Design review of the part built by this model. Coordinates are the model's own, in mm. Face numbers are marked on the shaded views. A direction names the side the tool comes from. Give positions to 0.01 mm unless a question says otherwise; leave off trailing zeros. Loops run counter-clockwise (first coordinate to the right, second up) from the corner with the lowest first, then second, coordinate; pieces in that order, holes last. Notation, with made-up numbers: (-4, -32) - (48, -32) arc R18 cw to (48, 0) - close; hole circle Ø6 at (-15.5, -37.75). An arc over 180 degrees is marked (long way). Write each question's results on one line, items separated by ' | '.
Autodesk Inventor part; units mm, degrees
ref_plane "YZ Plane" through (0, 0, 0) normal (1, 0, 0) x (0, 1, 0)
ref_plane "XZ Plane" through (0, 0, 0) normal (0, 1, 0) x (-1, 0, 0)
ref_plane "XY Plane" through (0, 0, 0) normal (0, 0, 1) x (1, 0, 0)
sketch "Sketch1" plane through (0, 0, 0) normal (0, 1, 0) x (-1, 0, 0)
  line L0 (0, 0) -> (127, 0)
  line L1 (127, 0) -> (127, 118.999)
  line L2 (127, 118.999) -> (0, 118.999)
  line L3 (0, 118.999) -> (0, 0)
  dimension "d0" = 127
  dimension "d1" = 118.999
extrude "Plate1" add sketch "Sketch1" along normal blind 3.048
sketch "Sketch2" plane through (-123.952, 0, 118.999) normal (-1, 0, 0) x (0, -1, 0)
  line L0 (0, -118.999) -> (0, 0)
  line L1 (0, 0) -> (-25.4, 0)
  line L2 (-25.4, 0) -> (-25.4, -118.999)
  line L3 (-25.4, -118.999) -> (0, -118.999)
edge flange "Flange1" height 25.4 angle 90 thickness 3.048 bend radius 3.048 thickness toward (-1, 0, 0) relief tear relief width 3.048 relief depth 1.524 edges at (-127, 3.048, 59.4995) wall of the first edge with corners at (-123.952, 0, 0) (-123.952, 0, 118.999) (-123.952, 25.4, 118.999) (-123.952, 25.4, 0)
bend "Bend1"
corner "Corner1"
sketch "Sketch3" plane through (-3.048, 0, 0) normal (1, 0, 0) x (0, 1, 0)
  line L0 (0, 118.999) -> (0, 0)
  line L1 (0, 0) -> (25.4, 0)
  line L2 (25.4, 0) -> (25.4, 118.999)
  line L3 (25.4, 118.999) -> (0, 118.999)
edge flange "Flange2" height 25.4 angle 90 thickness 3.048 bend radius 3.048 thickness toward (1, 0, 0) relief tear relief width 3.048 relief depth 1.524 edges at (0, 3.048, 59.4995) wall of the first edge with corners at (-3.048, 0, 118.999) (-3.048, 0, 0) (-3.048, 25.4, 0) (-3.048, 25.4, 118.999)
bend "Bend2"
corner "Corner2"
sketch "Sketch4" plane through (0, 3.048, 0) normal (0, 1, 0) x (1, 0, 0)
  line L0 (-120.904, 0) -> (-6.096, 0)
  line L1 (-6.096, -118.999) -> (-120.904, -118.999)
  point P0 (0, 0)
  point P1 (-63.5, -99.949)
  point P2 (-63.5, -19.05)
  dimension "d23" = 19.05
  dimension "d24" = 19.05
hole "Hole1" at (-63.5, 3.048, 99.949) at (-63.5, 3.048, 19.05) direction (0, -1, 0) diameter 6.35 end through all
sketch "Sketch5" plane through (-127, 25.4, 0) normal (-1, 0, 0) x (0, 0, 1)
  line L0 (118.999, 0) -> (118.999, -19.304)
  line L1 (0, -19.304) -> (0, 0)
  line L2 (118.999, -25.4) -> (0, -25.4)
  point P0 (7.112, -12.7)
  point P1 (111.887, -12.7)
  dimension "d32" = 7.112
  dimension "d33" = 7.112
  dimension "d34" = 12.7
  dimension "d35" = 12.7
hole "Hole2" at (-127, 12.7, 7.112) at (-127, 12.7, 111.887) direction (1, 0, 0) diameter 4.2926 depth 1016 tip angle 118
equation "\"d30\" = Thickness"
equation "\"d3\" = BendReliefWidth"
equation "\"d4\" = BendReliefDepth"
equation "\"d5\" = MinimumRemnant"
equation "\"d6\" = BendRadius"
equation "\"d9\" = BendRadius"
equation "\"d10\" = CornerReliefSize"
equation "\"d11\" = GapSize"
equation "\"d12\" = JacobiRadiusSize"
equation "\"d13\" = BendReliefWidth"
equation "\"d14\" = BendReliefDepth"
equation "\"d15\" = MinimumRemnant"
equation "\"d16\" = BendRadius"
equation "\"d19\" = BendRadius"
equation "\"d20\" = CornerReliefSize"
equation "\"d21\" = GapSize"
equation "\"d22\" = JacobiRadiusSize"
equation "\"BendRadius\" = Thickness"
equation "\"BendReliefWidth\" = Thickness"
equation "\"BendReliefDepth\" = 0.5 * Thickness"
equation "\"CornerReliefSize\" = 4 * Thickness"
equation "\"MinimumRemnant\" = 2 * Thickness"
equation "\"TransitionRadius\" = BendRadius"
equation "\"JacobiRadiusSize\" = BendRadius"
equation "\"GapSize\" = Thickness"
equation "\"d2\" = BendRadius"
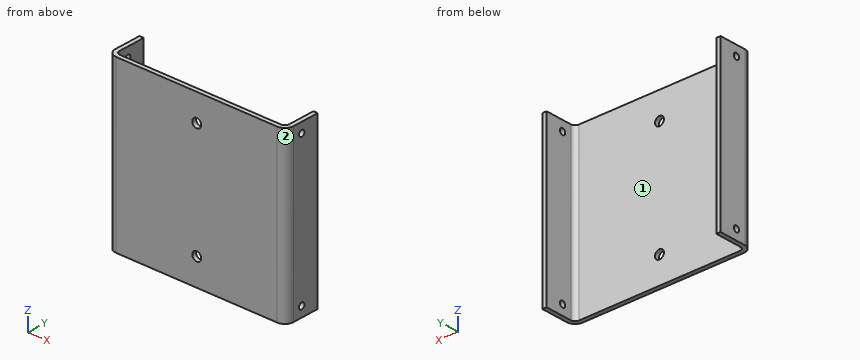
(1) Wall thickness on line 1 along Z through (x, y) = (-0.8, 12.7); line 2 along Z through (x, y) = (-63.5, 1.05) (3 decimals); line 3 along X through (y, z) = (14.75, 100.5): over which ranges is each line inside the solid? List them lowest first. Write a range as from..to.
Answers below:
line 1: 0..4.97, 9.26..109.74, 114.03..119 | line 2: 0..15.875, 22.225..96.774, 103.124..118.999 | line 3: -127..-123.95, -3.05..0
(2) Take a section at B-B on x = -63.5. Give the boundary of the cut face in (y, z) (3 decimals), plus the area to 3 significant figures.
Answers below:
outline: (0, 0) - (3.048, 0) - (3.048, 15.875) - (0, 15.875) - close; (0, 22.225) - (3.048, 22.225) - (3.048, 96.774) - (0, 96.774) - close; (0, 103.124) - (3.048, 103.124) - (3.048, 118.999) - (0, 118.999) - close | area: 324 mm2
(3) Take a section at A-A on y = 20.75. Give the boundary of the cut face in (x, z), plus the area to 3 significant figures.
Answers below:
outline: (-127, 0) - (-123.95, 0) - (-123.95, 119) - (-127, 119) - close; (-3.05, 0) - (0, 0) - (0, 119) - (-3.05, 119) - close | area: 725 mm2
(4) Tool access review of the marked faces 1 and 2: name each direction out of +Z, -Z, +X, -X, +Y, -Y from which nothing blocks a thin tool from reaching the whole face with its end or side.
Answers below:
face 1: +Z, -Z, +Y | face 2: +Z, -Z, +X, -Y
(5) Take a section at C-C on z = 19.05. Give the boundary of the cut face in (x, y) (3 decimals), plus the area to 3 significant figures.
Answers below:
outline: (-127, 6.096) arc R6.096 ccw to (-120.904, 0) - (-66.675, 0) - (-66.675, 3.048) - (-120.904, 3.048) arc R3.048 cw to (-123.952, 6.096) - (-123.952, 25.4) - (-127, 25.4) - close; (-60.325, 0) - (-6.096, 0) arc R6.096 ccw to (0, 6.096) - (0, 25.4) - (-3.048, 25.4) - (-3.048, 6.096) arc R3.048 cw to (-6.096, 3.048) - (-60.325, 3.048) - close | area: 492 mm2
(6) Insertion check: P1, Ø8, axis at y = 19.5, z = 57, coming from the +X side. The pin has a flat end and moves straight along its axis. Give the tip position at first contact, or say it passes through.
Answers below:
P1: x = 0
(7) Take a section at D-D on y = 12.7. Give the boundary of the cut face in (x, z).
Answers below:
outline: (-127, 0) - (-123.95, 0) - (-123.95, 4.97) - (-127, 4.97) - close; (-127, 9.26) - (-123.95, 9.26) - (-123.95, 109.74) - (-127, 109.74) - close; (-127, 114.03) - (-123.95, 114.03) - (-123.95, 119) - (-127, 119) - close; (-3.05, 0) - (0, 0) - (0, 4.97) - (-3.05, 4.97) - close; (-3.05, 9.26) - (0, 9.26) - (0, 109.74) - (-3.05, 109.74) - close; (-3.05, 114.03) - (0, 114.03) - (0, 119) - (-3.05, 119) - close
